Build history of the part. All positions in model axes, mm. Give positions to 0.01 mm unless a question says otherwise; leave off trailing zeros. Use one line per item in the form item = value. Start each with the question number.
Autodesk Inventor part; units mm, degrees
ref_plane "YZ Plane" through (0, 0, 0) normal (1, 0, 0) x (0, 1, 0)
ref_plane "XZ Plane" through (0, 0, 0) normal (0, 1, 0) x (-1, 0, 0)
ref_plane "XY Plane" through (0, 0, 0) normal (0, 0, 1) x (1, 0, 0)
sketch "Sketch1" plane through (0, 0, 0) normal (1, 0, 0) x (0, 1, 0)
  line L0 (18.6276, 30.145) -> (-681.3735, 30.145)
  line L1 (18.6276, 30.145) -> (18.6276, -29.8549)
  line L2 (18.6276, -29.8549) -> (-681.3735, -29.8549)
  line L3 (-681.3735, 30.145) -> (-1317.975, 30.145)
  line L4 (-1317.975, 30.145) -> (-1300.7166, -29.8549)
  line L5 (-1300.7166, -29.8549) -> (-681.3735, -29.8549)
  point P0 (0, 0)
  dimension "d0" = 700.0011
  dimension "d1" = 59.9999
extrude "Extrusion1" add sketch "Sketch1" along normal blind 150
sketch "Sketch2" plane through (0, 18.6276, 30.145) normal (0, 1, 0) x (1, 0, 0)
  line L0 (30.0948, 48.0392) -> (130.9532, 48.0392) construction
  line L1 (130.9532, 48.0392) -> (130.9532, 12.2508) construction
  line L2 (130.9532, 12.2508) -> (30.0948, 12.2508) construction
  line L3 (30.0948, 12.2508) -> (30.0948, 48.0392) construction
  point P0 (0, 30.145)
fillet "Fillet1" [suppressed]
chamfer "Chamfer1" [suppressed]
sketch "Sketch3" plane through (150, 18.6276, -29.8549) normal (0, 0, -1) x (-1, 0, 0)
  circle A0 centre (86.2337, -73.5365) radius 25.4
  circle A1 centre (86.2337, -207.3813) radius 25.4
  point P0 (150, -18.6276)
  dimension "d8" = 50.8
  dimension "d9" = 50.8
extrude "Extrusion2" cut sketch "Sketch3" against normal blind 150
fillet "Fillet2" radius 203.2 1 edges at (150, -1309.3458, 0.1451)
properties part number "legplate" material "Steel, High Strength, Low Alloy"
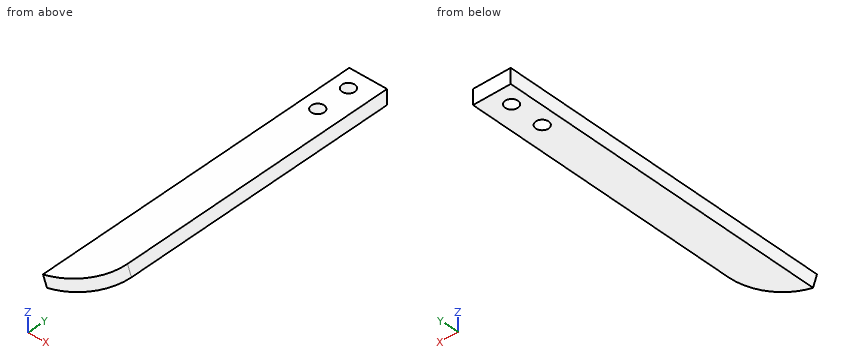
(1) Pin check, flat tip, straight feed: pin 1 Ø10 at (x, z) = (41.5, -7.5) entering from -Y. Stop position of the tip, or through.
(2) Cut at A-A, the plane z = 18. State how many separate pieces and enclosed holes the cut face has, then the cut area to 3 significant figures.
(3) Wall check: line 1 (Y direction, x = 61, z = -14.5); line 2 (Y direction, x = 43.5, z = -13); line 3 (Y direction, x = 10.5, z = -19). Give the ranges that are in metal, low to high. Write a range as from..to.
Solution:
q1.pin_1 = -1293.18
q2.separate_pieces = 1
q2.enclosed_holes = 2
q2.area = 188,000 mm2
q3.line_1 = -1275.96..-214, -163.5..-80.16, -29.66..18.63
q3.line_2 = -1287.46..-204.07, -173.44..-70.22, -39.6..18.63
q3.line_3 = -1300.56..18.63
